The listing builds one solid part. Answer for the finished solid, in the listing's coordinates (mm). Face numbers are marked on the shaded views. A direction names the side the tool comes from. Give positions to 0.01 mm unless a question says otherwise; leave off trailing zeros. Order: outer loops, then holes, each group sorted by start corner. A loop starts at its lowest first (then second) coordinate and runs counter-clockwise, first axis right, second up. Notation, with made-up numbers: (56, -29.5) - (111, -29.5) arc R24 ccw to (111, -14.5) - close; hole circle Ø3 at (76, 87.5). An arc over 180 degrees is marked (long way). Answer as a JSON object with one key per item and string values. Group by question number.
Q1. For the marked faces 1 and 2, determine the directions among +Z, -Z, +X, -X, +Y, -Y from which every point of the face is accessible in a straight line to the end or side of a thin tool.
Q2. A cutting plane is placed at C-C, the plane y = 7.75. Give the vertices of the cut face in (x, z), and give its area (3 significant figures).
Q3. A cutting plane is placed at B-B, the plane z = 18.75. Give the vertices of the cut face in (x, y).
Q4. Consider line 1 (Y direction, x = -23.5, z = 20.95); line 2 (X direction, y = 1.5, z = 16.5); line 3 (Z direction, x = 1, y = -3.75). Determine where each line is inside the solid, lowest interval first.
Q5. A cutting plane is placed at D-D, the plane x = 23.5. Give the vertices of the cut face in (y, z).
Q6. Given pin 1 (0.8 mm diameter, centred on x = -23.5, y = 11.5, fed in from +Z), flat-ended and moving along its own axis, determine where the tip first touches the part or whether it passes through.
Q7. A cutting plane is placed at A-A, the plane z = 11. Give the vertices of the cut face in (x, y).
from build123d import *

# Parameters (mm, degrees)
SKETCH_W     = 52
SKETCH_H     = 29
PAD_DEPTH    = 2
SKETCH001_W  = 5
SKETCH001_H  = 29
PAD001_DEPTH = 20
SKETCH002_R  = 0.75
POCKET_DEPTH = 5


with BuildPart() as part:
    # Sketch → Pad (new body)
    with BuildSketch(Plane.XY):
        Rectangle(SKETCH_W, SKETCH_H)
    extrude(amount=PAD_DEPTH)

    # Sketch001 (on Face6 of Pad) → Pad001 (join)
    with BuildSketch(Plane.XY.offset(2)):
        with Locations((-23.5, 0)):
            Rectangle(SKETCH001_W, SKETCH001_H)
        with Locations((23.5, 0)):
            Rectangle(SKETCH001_W, SKETCH001_H)
    extrude(amount=PAD001_DEPTH)

    # Sketch002 (on Face12 of Pad001) → Pocket (cut)
    with BuildSketch(Plane.XY.offset(22)):
        with Locations((-23.5, 11.75)):
            Circle(SKETCH002_R)
        with Locations((-23.5, -11.75)):
            Circle(SKETCH002_R)
        with Locations((23.5, 11.75)):
            Circle(SKETCH002_R)
        with Locations((23.5, -11.75)):
            Circle(SKETCH002_R)
    extrude(amount=-POCKET_DEPTH, mode=Mode.SUBTRACT)


solid = part.part
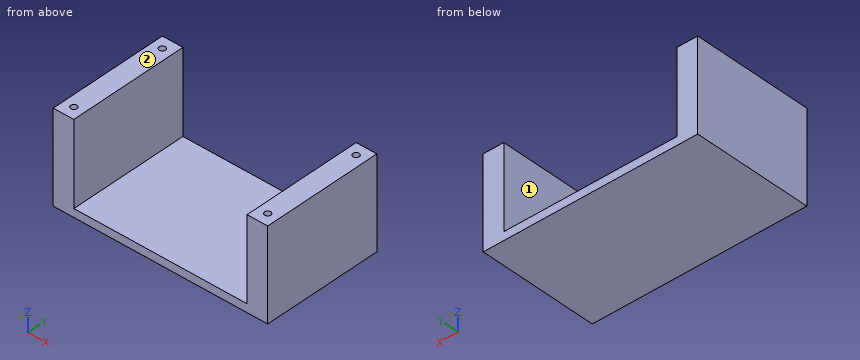
Reply:
{
 "1": {"face 1": "+Z, +Y, -Y", "face 2": "+Z, +X, -X, +Y, -Y"},
 "2": {"outline": "(-26, 0) - (26, 0) - (26, 22) - (21, 22) - (21, 2) - (-21, 2) - (-21, 22) - (-26, 22) - close", "area": "304 mm^2"},
 "3": {"outline": "(-26, -14.5) - (-21, -14.5) - (-21, 14.5) - (-26, 14.5) - close; (21, -14.5) - (26, -14.5) - (26, 14.5) - (21, 14.5) - close; hole circle Ø1.5 at (-23.5, -11.75); hole circle Ø1.5 at (-23.5, 11.75); hole circle Ø1.5 at (23.5, -11.75); hole circle Ø1.5 at (23.5, 11.75)"},
 "4": {"line 1": "y = -14.5 to -12.5, -11 to 11, 12.5 to 14.5", "line 2": "x = -26 to -21, 21 to 26", "line 3": "z = 0 to 2"},
 "5": {"outline": "(-14.5, 0) - (14.5, 0) - (14.5, 22) - (12.5, 22) - (12.5, 17) - (11, 17) - (11, 22) - (-11, 22) - (-11, 17) - (-12.5, 17) - (-12.5, 22) - (-14.5, 22) - close"},
 "6": {"pin 1": "stops at z = 17"},
 "7": {"outline": "(-26, -14.5) - (-21, -14.5) - (-21, 14.5) - (-26, 14.5) - close; (21, -14.5) - (26, -14.5) - (26, 14.5) - (21, 14.5) - close"}
}
